Geometry check sheet. Reference: the model listing, model coordinates, mm. Face numbers are marked on the shaded views. Give positions to 0.01 mm unless a question says otherwise; leave off trailing zeros. Write each loop counter-clockwise with the first axis right and the second up, starting at its lowest first coordinate (ties: lowest second). Pieces come first, ordered by that corner, then holes. Notation, with made-up numbers: (-29, -30) -> (7, -30) arc R35 cw to (7, 8) -> close; hole circle Ø8 at (7, 57.25). An arc over 180 degrees is marked (long way). Write item = value, one per line. Start each with the question number.
1. Mould release check, pull along X, two halves, no side actions. Record for the marked faces 1 and 2: pulls with the +X half, pulls with the -X half, needs draft (parallel to the pull), parting line crosses it, or undercut.
2. Cross-section at B-B, the plane z = -8. Record the cut outline in (x, y).
3. Thickness scan on line 1 along Y through (x, z) = (-14.5, 0); line 2 along X through (y, z) = (67, 0); line 3 along X through (y, z) = (202, 6). Record the ranges inside material, lowest first.
4. Cross-section at C-C, the plane y = 220. Record the cut outline in (x, z).
5. Depth check by flat-ended pin: P1, Ø6, axis at x = 11.5, z = -2, coming from the -Y side; P2, Ø1.5, axis at y = 213, z = 3.5, coming from the -X side; P3, Ø1.5, axis at x = -2.5, y = 63.5, coming from the +Z side; P4, Ø2.5, axis at y = 263, z = 0, coming from the +X side. Enter the tip coordinate at first touch or a pass-through.
6. Cross-section at A-A, the plane x = 8.5. Record the cut outline in (y, z).
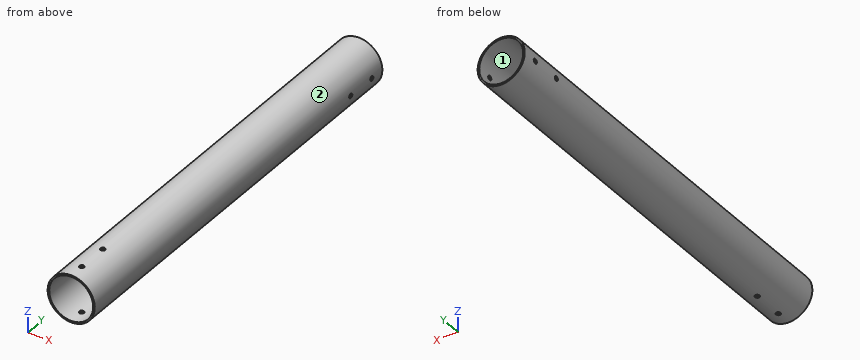
```python
from build123d import *

# Parameters (mm, degrees)
SKETCH_1_R               = 15
EXTRUDE_1_DEPTH          = 273
CUT_EXTRUDE_1_DEPTH      = 274.822935489
CUT_EXTRUDE_1_DEPTH_BACK = 274.822935489
SKETCH_2_R               = 1.5
CUT_EXTRUDE_2_DEPTH      = 274.8229356
CUT_EXTRUDE_2_DEPTH_BACK = 274.8229356
SKETCH_3_R               = 1.5
CUT_EXTRUDE_3_REACH      = 275.823
SKETCH_4_R               = 14


with BuildPart() as part:
    # 草圖1 → 填料-伸長1 (new body)
    with BuildSketch(Plane(origin=(0, 0, 0), x_dir=(1, 0, 0), z_dir=(0, 1, 0))):
        with Locations(Location((0, 0, 0), (0, 0, 270))):
            Circle(SKETCH_1_R)
    extrude(amount=EXTRUDE_1_DEPTH)

    # 草圖2 → 除料-伸長1 (cut, two sides: drawn at the far end of the back side and taken through both)
    with BuildSketch(Plane.XY.offset(-CUT_EXTRUDE_1_DEPTH_BACK)):
        with Locations((0, 10)):
            Circle(SKETCH_2_R)
        with Locations((0, 30)):
            Circle(SKETCH_2_R)
    extrude(amount=CUT_EXTRUDE_1_DEPTH + CUT_EXTRUDE_1_DEPTH_BACK, mode=Mode.SUBTRACT)

    # 草圖3 → 除料-伸長2 (cut, two sides: drawn at the far end of the back side and taken through both)
    with BuildSketch(Plane(origin=(0, 0, 0), x_dir=(0, 0, -1), z_dir=(1, 0, 0)).offset(-CUT_EXTRUDE_2_DEPTH_BACK)):
        with Locations((0, 263)):
            Circle(SKETCH_3_R)
        with Locations((0, 243)):
            Circle(SKETCH_3_R)
    extrude(amount=CUT_EXTRUDE_2_DEPTH + CUT_EXTRUDE_2_DEPTH_BACK, mode=Mode.SUBTRACT)

    # 草圖4 → 除料-伸長3 (cut, up to next)
    with BuildSketch(Plane(origin=(0, 273, 0), x_dir=(1, 0, 0), z_dir=(0, 1, 0)), mode=Mode.PRIVATE) as cut_extrude_3_sk1:
        with Locations(Location((0, 0, 0), (0, 0, 270))):
            Circle(SKETCH_4_R)
    cut_extrude_3_tool1 = extrude(cut_extrude_3_sk1.sketch, amount=-CUT_EXTRUDE_3_REACH, mode=Mode.PRIVATE) & part.part
    add(cut_extrude_3_tool1.solids().sort_by_distance((0, 273, 0))[0], mode=Mode.SUBTRACT)


solid = part.part
```
Answers:
q1.face_1 = undercut
q1.face_2 = parting line crosses it
q2.outline = (-12.69, 0) -> (-11.49, 0) -> (-11.49, 273) -> (-12.69, 273) -> close; (11.49, 0) -> (12.69, 0) -> (12.69, 273) -> (11.49, 273) -> close
q3.line_1 = 0 to 241.5, 244.5 to 261.5, 264.5 to 273
q3.line_2 = -15 to -14, 14 to 15
q3.line_3 = -13.75 to -12.65, 12.65 to 13.75
q4.outline = circle Ø30 at (0, 0); hole circle Ø28 at (0, 0)
q5.P1 = 0
q5.P2 = -14.75
q5.P3 = 14.9
q5.P4 = through
q6.outline = (0, -12.36) -> (273, -12.36) -> (273, -11.12) -> (0, -11.12) -> close; (0, 11.12) -> (273, 11.12) -> (273, 12.36) -> (0, 12.36) -> close
